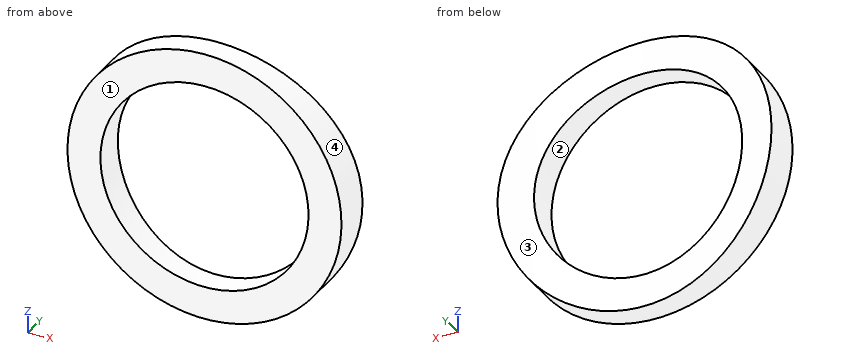
from build123d import *

# Parameters (mm, degrees)
SKETCH1_R                = 10.4
SKETCH1_R_2              = 7.9
BOSS_EXTRUDE1_DEPTH      = 3.2
SURFACE_EXTRUDE1_1_BACK  = 15
SURFACE_EXTRUDE1_1_DEPTH = 30


with BuildPart() as part:
    # Sketch1 → Boss-Extrude1 (new body)
    with BuildSketch(Plane(origin=(0, 0, 0), x_dir=(1, 0, 0), z_dir=(0, 1, 0))):
        with Locations(Location((0, 0, 0), (0, 0, 270))):
            Circle(SKETCH1_R)
        with Locations(Location((0, 0, 0), (0, 0, 270))):
            Circle(SKETCH1_R_2, mode=Mode.SUBTRACT)
    extrude(amount=BOSS_EXTRUDE1_DEPTH)

    # SurfaceCut5: cut with a surface, the side behind it stays
    # Surface-Extrude1: a surface, the sketch's curves swept straight by 30 mm
    with BuildLine(Plane.XY.offset(-SURFACE_EXTRUDE1_1_BACK), mode=Mode.PRIVATE) as surface_extrude1_1_path:
        CenterArc((0, 46.25), 44.45, 0, 360)
    surface_extrude1_1 = Shell.extrude(surface_extrude1_1_path.wire(), (0 * SURFACE_EXTRUDE1_1_DEPTH, 0 * SURFACE_EXTRUDE1_1_DEPTH, 1 * SURFACE_EXTRUDE1_1_DEPTH))
    split(bisect_by=surface_extrude1_1, keep=Keep.BOTTOM)


solid = part.part
The listing builds one solid part. Answer for the finished solid, in the listing's coordinates (mm). Face numbers are marked on the shaded views. Coordinates: 2 decimals unless noted, no trailing zeros. Loops run counter-clockwise (first coordinate to the right, second up) from the corner with the lowest first, then second, coordinate; pieces in that order, holes last.
1) Find section B-B on z = 0. Write down the section's boundary in (x, y), then the cut area to 3 significant figures.
2) Find section C-C on x = 9. Write down the section's boundary in (y, z).
3) Flat-ended cylindrical pins translate along their axes: pin 1 Ø1 at (y, z) = (2.5, -2) entering from +X; pin 2 Ø1.5 at (y, z) = (2, -1.5) entering from -X; pin 3 Ø1 at (x, z) = (7.5, -2.5) entering from -Y. Find the tip coordinate at first contact, or state that the pin passes through.
4) Determine the mould class of the marked faces 1, 2, 3 and 4 for opening direction X: pulls with the +X half, pulls with the -X half, needs draft (parallel to the pull), parting line crosses it, or undercut.
5) Find the intervals of material crossed by L1, parallel to Z at x = 0, y = 0.95; L2, parallel to Z at x = 2.5, y = 0.8, in increasing order.
6) Find section A-A on x = 0. Write down the section's boundary in (y, z), then the cut area to 3 significant figures.
Values:
1. outline: (-10.4, 0) - (-7.9, 0) - (-7.9, 2.51) arc R44.45 cw to (-10.4, 3.03) - close; (7.9, 0) - (10.4, 0) - (10.4, 3.03) arc R44.45 cw to (7.9, 2.51) - close
1. area: 13.8 mm2
2. outline: (0, -5.21) - (2.72, -5.21) - (2.72, 5.21) - (0, 5.21) - close
3. pin 1: stops at x = 10.29
3. pin 2: stops at x = -10.37
3. pin 3: stops at y = 0
4. face 1: needs draft
4. face 2: undercut
4. face 3: undercut
4. face 4: parting line crosses it
5. L1: z = -10.4 to -7.9, 7.9 to 10.4
5. L2: z = -10.1 to -7.49, 7.49 to 10.1
6. outline: (0, -10.4) - (1.8, -10.4) - (1.8, -7.9) - (0, -7.9) - close; (0, 7.9) - (1.8, 7.9) - (1.8, 10.4) - (0, 10.4) - close
6. area: 9.00 mm2
